Build history of the part. All positions in model axes, mm. A direction names the side the tool comes from. Give positions to 0.01 mm unless a question says otherwise; leave off trailing zeros. Write each loop counter-clockwise with the first axis right and the second up, starting at its lowest first coordinate (ties: lowest second). Pieces come first, ordered by that corner, then holes. Notation, with made-up numbers: (-25, 26) -> (-1, 26) arc R15 cw to (-1, 35) -> close; hole circle Ø3 at (-15, -23.5). An arc over 180 degrees is marked (long way). Write item = value, one per line. Start each with the question number.
Q1. Saw through at A-A, the plane z = 140. List the corners of the cut face in (x, y), then the cut area to 3 significant figures.
Q2. Mould opens along Y. For faces 3 (the face through (4, -3, 19)), 4 (the face through (23, -50, 132)), 5 (the face through (23, 50, 132)), 6 (the face through (6.307, 38.792, 132.786)) say: pulls with the +Y half, pulls with the -Y half, needs draft (parallel to the pull), parting line crosses it, or undercut.
Q3. Wall check: line 1 (Y direction, x = 11, z = 248); line 2 (X direction, y = -29.5, z = 199.5); line 3 (Y direction, x = 22, z = 266). Give the ranges that are in metal, low to high.
Q4. Saw through at D-D, the plane x = 8. List the corners of the cut face in (y, z).
Q5. Saw through at B-B, the plane x = 33.5. List the corners of the cut face in (y, z).
Q6. Drop a flat-ended pin along its axis: P1, Ø8, axis at y = 18.5, z = 212.5, coming from the +X side. Give the stop position or say it passes through.
Q7. Tool access for faces 1 (the face through (4.5, 0, 133)), 2 (the face through (0, -1, 133)): list every direction of +Z, -Z, +X, -X, +Y, -Y with a clear straight run to the whole face (end or side of a thin tool).
Q8. Saw through at C-C, the plane y = -2. List the corners of the cut face in (x, z), then the cut area to 3 significant figures.
Autodesk Inventor part; units mm, degrees
ref_plane "Начальная плоскость" through (0, 0, -23) normal (0, 0, 1) x (1, 0, 0)
ref_plane "Конечная плоскость" through (0, 0, 292) normal (0, 0, 1) x (1, 0, 0)
ref_plane "РабПлоскость8" through (46, 0, 292) normal (-0.7071, 0, 0.7071) x (0.7071, 0, 0.7071)
ref_plane "Начальная плоскость" through (0, 0, -23) normal (0, 0, 1) x (1, 0, 0)
ref_plane "Конечная плоскость" through (0, 0, 292) normal (0, 0, 1) x (1, 0, 0)
sketch "Эскиз" plane through (0, 0, 0) normal (0, 0, 1) x (1, 0, 0)
  line L0 (46, -50) -> (0, -50)
  line L1 (46, -50) -> (46, -46.6496)
  line L2 (43.2392, -43.6591) -> (10.9418, -41.0753)
  line L3 (4.5, -34.0976) -> (4.5, 34.0976)
  line L4 (43.2392, 43.6591) -> (10.9418, 41.0753)
  line L5 (46, 46.6496) -> (46, 50)
  line L6 (0, 50) -> (46, 50)
  line L7 (0, -50) -> (0, 50)
  arc A0 (4.5, -34.0976) -> (10.9418, -41.0753) centre (11.5, -34.0976) ccw
  arc A1 (10.9418, 41.0753) -> (4.5, 34.0976) centre (11.5, 34.0976) ccw
  arc A2 (46, -46.6496) -> (43.2392, -43.6591) centre (43, -46.6496) ccw
  arc A3 (43.2392, 43.6591) -> (46, 46.6496) centre (43, 46.6496) ccw
  line L8 (0, 70) -> (0, -70) construction
  line L9 (-9.3169, 0) -> (55.9016, 0) construction
  point P0 (46, -43.88)
  point P1 (4.5, -40.56)
  point P2 (4.5, 40.56)
  point P3 (46, 43.88)
  dimension "d3" = 46
  dimension "d5" = 4.5
  dimension "d7" = 100
  dimension "d9" = 9.44
  dimension "d11" = 9.44
  dimension "d13" = 6.12
  dimension "d15" = 6.12
  dimension "d22" = 7
  dimension "d23" = 3
  dimension "d24" = 50
  dimension "d25" = 0
extrude "Тело" add sketch "Эскиз" along normal up to surface (315 mm away) from surface at -23
sketch "Sketch3" plane through (0, 0, 0) normal (0, 0, 1) x (1, 0, 0)
  line L0 (0, 0) -> (10, 0)
ref_plane "Work Plane7" through (0, 0, 0) normal (0, -1, 0) x (1, 0, 0)
sketch "Sketch4" plane through (0, 0, 0) normal (0, -1, 0) x (1, 0, 0)
  line L0 (-2, -23) -> (12, -23)
  line L1 (-2, 292) -> (12, 292)
  dimension "d29" = 315
ref_plane "РабПлоскость8" through (46, 0, 292) normal (-0.7071, 0, 0.7071) x (0.7071, 0, 0.7071)
split "Разделение1" plane through (46, 0, 292) removes the side toward (-0.7071, 0, 0.7071)
ref_plane "РабПлоскость9" through (46, 0, -23) normal (-0.7071, 0, -0.7071) x (-0.7071, 0, 0.7071)
split "Разделение2" plane through (46, 0, -23) removes the side toward (-0.7071, 0, -0.7071)
equation "\"d3\" = b"
equation "\"d7\" = ParH"
equation "\"d22\" = R"
equation "\"d23\" = R1"
equation "\"d24\" = 0.5 * d7"
equation "\"d16\" = G_L"
equation "\"R1\" = 3"
equation "\"R\" = 7"
equation "\"t1\" = 4.5"
equation "\"t2\" = 7.6"
equation "\"ParH\" = 100"
equation "\"b\" = 46"
equation "\"msp_x1\" = 0.04 * b"
equation "\"msp_x2\" = -0.08 * t1 + 0.04 * b"
equation "\"G_L\" = d29"
equation "\"ex\" = 0"
equation "\"G_OFFSET_START\" = 23"
equation "\"G_OFFSET_END\" = 23"
equation "\"d26\" = -G_OFFSET_START"
equation "\"d27\" = G_OFFSET_END + B_L"
equation "\"B_L\" = 269"
properties part number "Швеллер 10U-315 ГОСТ 8240-97" material "Сталь, мягкая"
Report:
q1.outline = (0, -50) -> (46, -50) -> (46, -46.65) arc R3 ccw to (43.24, -43.66) -> (10.94, -41.08) arc R7 cw to (4.5, -34.1) -> (4.5, 34.1) arc R7 cw to (10.94, 41.08) -> (43.24, 43.66) arc R3 ccw to (46, 46.65) -> (46, 50) -> (0, 50) -> close
q1.area = 1,110 mm2
q2.face_3 = needs draft
q2.face_4 = pulls with the -Y half
q2.face_5 = pulls with the +Y half
q2.face_6 = undercut
q3.line_1 = -50 to -41.08, 41.08 to 50
q3.line_2 = 0 to 4.5
q3.line_3 = -50 to -41.96, 41.96 to 50
q4.outline = (-50, 15) -> (-40.16, 15) -> (-40.16, 254) -> (-50, 254) -> close; (40.16, 15) -> (50, 15) -> (50, 254) -> (40.16, 254) -> close
q5.outline = (-50, -10.5) -> (-42.88, -10.5) -> (-42.88, 279.5) -> (-50, 279.5) -> close; (42.88, -10.5) -> (50, -10.5) -> (50, 279.5) -> (42.88, 279.5) -> close
q6.P1 = 4.5
q7.face_1 = +Z, -Z, +X
q7.face_2 = +Z, -Z, -X, +Y, -Y
q8.outline = (0, 23) -> (4.5, 18.5) -> (4.5, 250.5) -> (0, 246) -> close
q8.area = 1,020 mm2
